Autodesk Inventor part; units mm, degrees
ref_plane "YZ Plane" through (0, 0, 0) normal (1, 0, 0) x (0, 1, 0)
ref_plane "XZ Plane" through (0, 0, 0) normal (0, 1, 0) x (-1, 0, 0)
ref_plane "XY Plane" through (0, 0, 0) normal (0, 0, 1) x (1, 0, 0)
sketch "Sketch1" plane through (0, 0, 0) normal (0, 0, 1) x (1, 0, 0)
  line L0 (0, 107) -> (0, -103) construction
  line L1 (-117, 0) -> (116, 0) construction
  arc A0 (-38.3571, 10.8766) -> (-30.6918, -5.8614) centre (-40, 0) ccw
  arc A1 (30.6918, -5.8614) -> (38.3571, 10.8766) centre (40, 0) ccw
  arc A2 (40, 0) -> (-40, 0) centre (0, -69.282) ccw construction
  line L2 (-40, 13) -> (-40, -15) construction
  line L3 (40, 13) -> (40, -15) construction
  arc A3 (25.8036, -1.8505) -> (-25.8036, -1.8505) centre (0, -69.282) ccw
  arc A4 (33.0749, 11.5099) -> (-33.0749, 11.5099) centre (0, -69.282) ccw
  arc A5 (-38.3571, 10.8766) -> (-33.0749, 11.5099) centre (-36.8635, 20.7645) ccw
  arc A6 (-25.8036, -1.8505) -> (-30.6918, -5.8614) centre (-22.2297, -11.19) ccw
  arc A7 (33.0749, 11.5099) -> (38.3571, 10.8766) centre (36.8635, 20.7645) ccw
  arc A8 (30.6918, -5.8614) -> (25.8036, -1.8505) centre (22.2297, -11.19) ccw
  line L4 (-39.7655, 0.1354) -> (-60.5453, -11.8618) construction
  line L5 (-46.3958, 11.0778) -> (-33.6042, -11.0778) construction
  circle A9 centre (-43.75, 6.4952) radius 0.5
  circle A10 centre (-36.25, -6.4952) radius 0.5
  circle A11 centre (43.75, 6.4952) radius 0.5
  circle A12 centre (36.25, -6.4952) radius 0.5
  circle A13 centre (-40, 0) radius 3.5
  circle A14 centre (40, 0) radius 3.5
  point P0 (0, 0)
  dimension "d0" = 22
  dimension "d1" = 40
  dimension "d2" = 80
  dimension "d6" = 10
  dimension "d7" = 72.2
  dimension "d8" = 87.3
  dimension "d9" = 1
  dimension "d10" = 7.5
  dimension "d11" = 7
extrude "Extrusion1" add sketch "Sketch1" along normal blind 3
properties part number "Femur"
Geometry: final body of the model. Coordinates: model frame, mm. A direction names the side the tool comes from. Coordinates: 2 decimals unless noted, no trailing zeros. Write each loop counter-clockwise with the first axis right and the second up, starting at its lowest first coordinate (ties: lowest second). Pieces come first, ordered by that corner, then holes. Notation, with made-up numbers: M 58.5,42 L 85.5,42 A18 ccw 85.5,54 Z; hole C 66.5,46.25 d2. An arc over 180 degrees is marked long. Answer as CSV lines item,"result". Start each with the question number.
Q1. Pin query (flat end, axial travel): P1, Ø1, axis at y = -6.5, z = 2, coming from the +X side. Return the tip coordinate at first contact, or that it passes through.
Q2. Cut plane B-B on y = -5. Return the cut outline in (x, z).
Q3. Line query: line 1 (X direction, y = -2, z = 1.9); line 2 (X direction, y = 3, z = 1.3); line 3 (X direction, y = -2.5, z = 0.3). Output: solid intervals per line, ascending. Write a range as from..to.
Q4. Cut plane A-A on x = -40. Return the cut outline in (y, z).
Q5. Cut plane C-C on y = 0. Return the cut outline in (x, z).
Q6. Reachability of faces 4 (the cylindrical face through (28.5, -3.4, 1.5)), 5 (the flat face through (-1, 4, 3)) from +Z, -Z, +X, -X, +Y, -Y: full face, straight path, thin tool, end or side. Return the list, or none.
Q7. Mould query, pull axis X, two halves, no side actions, for faces 1 (the cylindrical face through (-0.475, 18.017, 1.479)), 2 (the cylindrical face through (-43.497, -0.154, 1.479)), 3 (the flat face through (-1, 4, 0)). Classes: released by +X, released by -X, zero draft, split by the parting line, or undercut.
Q8. Cut plane D-D on z = 2.1. Return the cut outline in (x, y).
Findings below:
1,P1,"stops at x = 49.22"
2,outline,"M -49.8,0 L -30.08,0 L -30.08,3 L -49.8,3 Z; M 30.08,0 L 49.8,0 L 49.8,3 L 30.08,3 Z"
3,line 1,"x = -50.82..-42.87, -37.13..-26.17, 26.17..37.13, 42.87..50.82"
3,line 2,"x = -50.58..-41.8, -38.2..38.2, 41.8..50.58"
3,line 3,"x = -50.71..-42.45, -37.55..-27.18, 27.18..37.55, 42.45..50.71"
4,outline,"M -11,0 L -3.5,0 L -3.5,3 L -11,3 Z; M 3.5,0 L 11,0 L 11,3 L 3.5,3 Z"
5,outline,"M -51,0 L -43.5,0 L -43.5,3 L -51,3 Z; M -36.5,0 L -20.32,0 L -20.32,3 L -36.5,3 Z; M 20.32,0 L 36.5,0 L 36.5,3 L 20.32,3 Z; M 43.5,0 L 51,0 L 51,3 L 43.5,3 Z"
6,face 4,"+Z, -Z, -Y"
6,face 5,"+Z, +X, -X, +Y, -Y"
7,face 1,"split by the parting line"
7,face 2,"undercut"
7,face 3,"zero draft"
8,outline,"M -38.36,10.88 A11 ccw long -30.69,-5.86 A10 cw -25.8,-1.85 A72.2 cw 25.8,-1.85 A10 cw 30.69,-5.86 A11 ccw long 38.36,10.88 A10 cw 33.07,11.51 A87.3 ccw -33.07,11.51 A10 cw Z; hole C -43.75,6.5 d1; hole C -40,0 d7; hole C -36.25,-6.5 d1; hole C 36.25,-6.5 d1; hole C 40,0 d7; hole C 43.75,6.5 d1"
